The listing builds one solid part. Answer for the finished solid, in the listing's coordinates (mm). A direction names the side the tool comes from. Coordinates: 2 decimals unless noted, no trailing zeros. Order: outer loops, then holes, each group sorted by start corner. A loop starts at its lowest first (then second) coordinate and runs counter-clockwise, first axis right, second up. Notation, with made-up numbers: (1, 51.25) -> (25, 51.25) arc R26 cw to (25, 82.25) -> close; hole circle Ø9 at (45.5, 0.25). An arc over 180 degrees is marked (long way). Answer in a Markdown table with one row per item. Add a question column.
```python
from build123d import *

# Parameters (mm, degrees)
SKETCH1_W           = 97
SKETCH1_H           = 130
BOSS_EXTRUDE1_DEPTH = 12
SKETCH9_R           = 21
SKETCH9_R_2         = 2
CUT_EXTRUDE2_DEPTH  = 12
SKETCH11_W          = 109
SKETCH11_H          = 142
SKETCH11_W_2        = 97
SKETCH11_H_2        = 130
BOSS_EXTRUDE4_DEPTH = 32
SKETCH18_W          = 20
SKETCH18_H          = 60
BOSS_EXTRUDE5_DEPTH = 3
SKETCH14_R          = 15
CUT_EXTRUDE5_DEPTH  = 134.962681371
SKETCH20_W          = 91
SKETCH20_H          = 20
BOSS_EXTRUDE6_DEPTH = 4
SKETCH21_R          = 2
CUT_EXTRUDE6_DEPTH  = 9


with BuildPart() as part:
    # Sketch1 → Boss-Extrude1 (new body)
    with BuildSketch(Plane.XY):
        Rectangle(SKETCH1_W, SKETCH1_H)
    extrude(amount=BOSS_EXTRUDE1_DEPTH)

    # Sketch9 → Cut-Extrude2 (cut)
    with BuildSketch(Plane.XY.offset(12)):
        with Locations((0, 18)):
            Circle(SKETCH9_R)
        with Locations((0, 44)):
            Circle(SKETCH9_R_2)
        with Locations((22.516660498, 31)):
            Circle(SKETCH9_R_2)
        with Locations((22.516660498, 5)):
            Circle(SKETCH9_R_2)
        with Locations((0, -8)):
            Circle(SKETCH9_R_2)
        with Locations((-22.516660498, 5)):
            Circle(SKETCH9_R_2)
        with Locations((-22.516660498, 31)):
            Circle(SKETCH9_R_2)
    extrude(amount=-CUT_EXTRUDE2_DEPTH, mode=Mode.SUBTRACT)

    # Sketch11 → Boss-Extrude4 (add)
    with BuildSketch(Plane.XY):
        Rectangle(SKETCH11_W, SKETCH11_H)
        Rectangle(SKETCH11_W_2, SKETCH11_H_2, mode=Mode.SUBTRACT)
    extrude(amount=BOSS_EXTRUDE4_DEPTH)

    # Sketch18 → Boss-Extrude5 (add)
    with BuildSketch(Plane(origin=(-48.5, 0, 0), x_dir=(0, 0, -1), z_dir=(1, 0, 0))):
        with Locations((-22, -35)):
            Rectangle(SKETCH18_W, SKETCH18_H)
    boss_extrude5 = extrude(amount=BOSS_EXTRUDE5_DEPTH)

    # Mirror1: Boss-Extrude5 across plane
    add(boss_extrude5.mirror(Plane(origin=(0, 0, 0), x_dir=(0, 0, 1), z_dir=(1, 0, 0))))

    # Sketch14 → Cut-Extrude5 (cut, through all)
    with BuildSketch(Plane.ZY.offset(54.5)):
        with Locations((32, -34)):
            Circle(SKETCH14_R)
    extrude(amount=-CUT_EXTRUDE5_DEPTH, mode=Mode.SUBTRACT)

    # Sketch20 → Boss-Extrude6 (add)
    with BuildSketch(Plane(origin=(0, -65, 0), x_dir=(1, 0, 0), z_dir=(0, 1, 0))):
        with Locations((0, -22)):
            Rectangle(SKETCH20_W, SKETCH20_H)
    extrude(amount=BOSS_EXTRUDE6_DEPTH)

    # Sketch21 → Cut-Extrude6 (cut)
    with BuildSketch(Plane.ZY.offset(54.5)):
        with Locations((32, -10)):
            Circle(SKETCH21_R)
        with Locations((8, -10)):
            Circle(SKETCH21_R)
        with Locations((56, -10)):
            Circle(SKETCH21_R)
        with Locations((56, -58)):
            Circle(SKETCH21_R)
        with Locations((32, -58)):
            Circle(SKETCH21_R)
        with Locations(Location((8, -58, 0), (0, 0, 180))):
            Circle(SKETCH21_R)
        with Locations((8, -34)):
            Circle(SKETCH21_R)
    cut_extrude6 = extrude(amount=-CUT_EXTRUDE6_DEPTH, mode=Mode.SUBTRACT)

    # Mirror2: Cut-Extrude6 across plane
    add(cut_extrude6.mirror(Plane(origin=(0, 0, 0), x_dir=(0, 0, 1), z_dir=(1, 0, 0))), mode=Mode.SUBTRACT)


solid = part.part
```
Q1. For faces 1 (the face through (47, -5, 22)), 2 (the face through (45.5, -10, 8)), 3 (the face through (12, 66, 32)), 4 (the face through (-45.5, -58, 8)), determine the directions among +Z, -Z, +X, -X, +Y, -Y from which every point of the face is accessible in a straight line to the end or side of a thin tool.
Q2. Determine the mould class of faces 5 (the face through (22.08, 29.05, 6.08)), 6 (the face through (-50, -16, 32)) for opening direction Y: +Y half, -Y half, draft (parallel to the pull), parting line (faces both ways), or undercut.
Q3. A cutting plane is placed at D-D (z = 28.5). Determine the outline of the cut face in (x, y).
Q4. Given pin 1 (3 mm diameter, centred on y = -10, z = 8, fed in from +X); pin 2 (6.5 mm diameter, centred on x = 22.52, y = 5, fed in from +Z); pin 3 (2.5 mm diameter, centred on y = -34, z = 8, fed in from -X), each flat-ended and moving along its own axis, determine where each tip first touches the part or whether it passes through.
Q5. A cutting plane is placed at B-B (x = 0). Determine the outline of the cut face in (y, z), then the cut area to 3 significant figures.
Q6. Straight lines are drawn through the part: line 1 (Y direction, x = 0, z = 3.5); line 2 (Y direction, x = -30.5, z = 25.5); line 3 (Y direction, x = 51, z = 8). For each, find the intervals that lie inside material, in ascending order.
Q7. A cutting plane is placed at A-A (y = 44). Determine the outline of the cut face in (x, z), then the cut area to 3 significant figures.
Q8. A cutting plane is placed at C-C (y = -58). Determine the outline of the cut face in (x, z).
Returned:
| question | item | result |
|---|---|---|
| 1 | face 1 | +Z |
| 1 | face 2 | +X |
| 1 | face 3 | +Z, +X, -X, +Y, -Y |
| 1 | face 4 | -X |
| 2 | face 5 | undercut |
| 2 | face 6 | draft |
| 3 | outline | (-54.5, -71) -> (54.5, -71) -> (54.5, -48.59) -> (45.5, -48.59) -> (45.5, -61) -> (-45.5, -61) -> (-45.5, -48.59) -> (-54.5, -48.59) -> close; (-54.5, -19.41) -> (-45.5, -19.41) -> (-45.5, -5) -> (-48.5, -5) -> (-48.5, 65) -> (48.5, 65) -> (48.5, -5) -> (45.5, -5) -> (45.5, -19.41) -> (54.5, -19.41) -> (54.5, 71) -> (-54.5, 71) -> close |
| 4 | pin 1 | stops at x = 45.5 |
| 4 | pin 2 | stops at z = 12 |
| 4 | pin 3 | stops at x = -45.5 |
| 5 | outline | (-71, 0) -> (-10, 0) -> (-10, 12) -> (-61, 12) -> (-61, 32) -> (-71, 32) -> close; (-6, 0) -> (-3, 0) -> (-3, 12) -> (-6, 12) -> close; (39, 0) -> (42, 0) -> (42, 12) -> (39, 12) -> close; (46, 0) -> (71, 0) -> (71, 32) -> (65, 32) -> (65, 12) -> (46, 12) -> close |
| 5 | area | 1,420 mm² |
| 6 | line 1 | y = -71 to -10, -6 to -3, 39 to 42, 46 to 71 |
| 6 | line 2 | y = -71 to -61, 65 to 71 |
| 6 | line 3 | y = -71 to -60, -56 to -36, -32 to -12, -8 to 71 |
| 7 | outline | (-54.5, 0) -> (-2, 0) -> (-2, 12) -> (-48.5, 12) -> (-48.5, 32) -> (-54.5, 32) -> close; (2, 0) -> (54.5, 0) -> (54.5, 32) -> (48.5, 32) -> (48.5, 12) -> (2, 12) -> close |
| 7 | area | 1,500 mm² |
| 8 | outline | (-54.5, 0) -> (54.5, 0) -> (54.5, 6) -> (45.5, 6) -> (45.5, 10) -> (54.5, 10) -> (54.5, 30) -> (45.5, 30) -> (45.5, 12) -> (-45.5, 12) -> (-45.5, 30) -> (-54.5, 30) -> (-54.5, 10) -> (-45.5, 10) -> (-45.5, 6) -> (-54.5, 6) -> close |
